Drawing for the job (mm, zero at the part's lowest x, y, z). A direction names the side the tool comes from. Coordinates: 2 decimals unless noted, no trailing zeros. Order: outer loops, then holes, each group sorted by start corner. A loop starts at its lowest first (then second) coordinate and runs counter-clockwise, first axis right, second up. Notation, with made-up numbers: (71, 72) - (114, 72) arc R19 cw to (114, 101) - close; hole circle Ø1 at (23, 44.25). An arc over 180 degrees is marked (long way). Put each result on its own line as item: value. Start each with the question number.
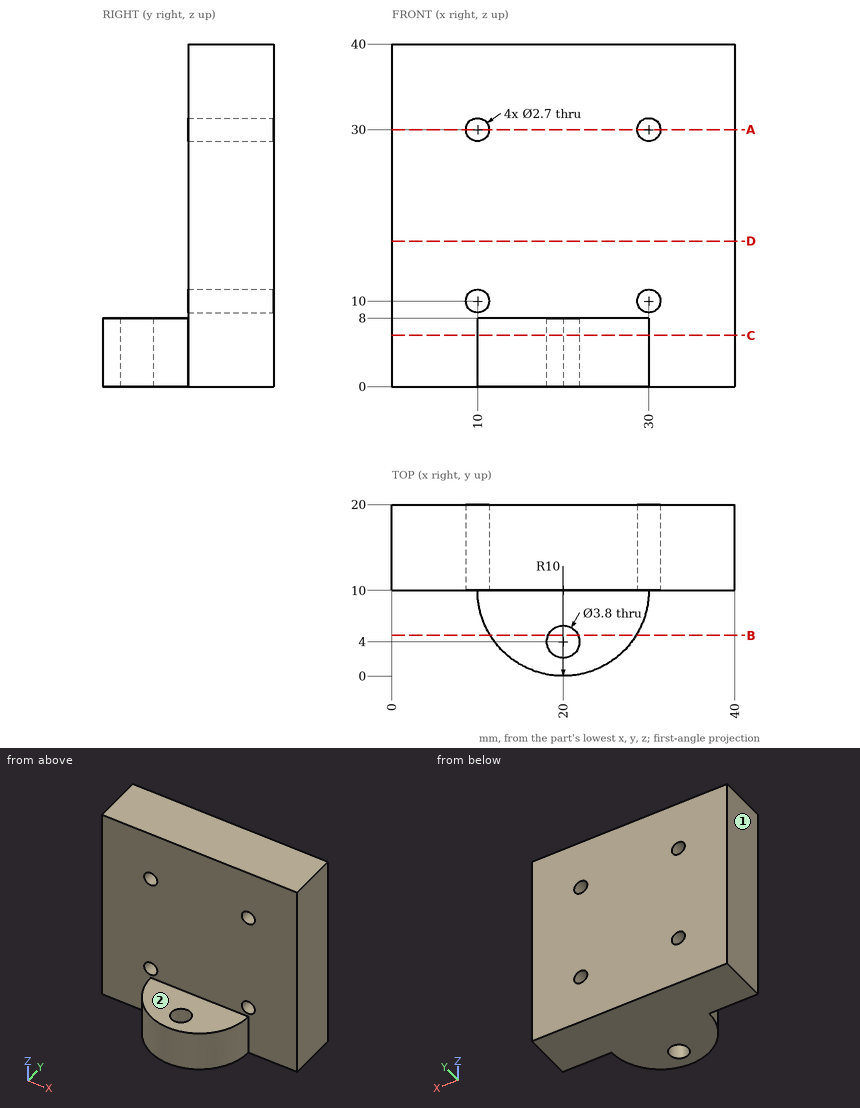
Item 1: Wall check: line 1 along X through (y, z) = (16.25, 30); line 2 along Y through (x, z) = (9, 3); line 3 along Z through (x, y) = (25, 9). Give the ranges that are in metal, low to high.
Item 2: Flat gauge pins, fed straight in: pin 1 Ø3 at (x, z) = (13, 34.5) entering from -Y; pin 2 Ø1.5 at (x, y) = (27, 3.5) entering from +Z. Where does each tip first touch, or does it go through?
Item 3: 3-axis set-ups, long thin cutter, end or side, ignore diameter. For the marked faces 1 and 2: which of +Z, -Z, +X, -X, +Y, -Y reach the whole face in a straight line?
Item 4: Slice it at D-D, the plane z = 17. Give the cut face in (x, y), plus the area to 3 significant figures.
Item 5: Slice it at B-B, the plane y = 4.75. Give the cut face in (x, z).
Item 6: Slice it at C-C, the plane z = 6. Give the cut face in (x, y), plus the area to 3 significant figures.
Item 7: Slice it at A-A, the plane z = 30. Give the cut face in (x, y), plus the area to 3 significant figures.
Here are the results:
1. line 1: x = 0 to 8.65, 11.35 to 28.65, 31.35 to 40
1. line 2: y = 10 to 20
1. line 3: z = 0 to 8
2. pin 1: stops at y = 10
2. pin 2: stops at z = 8
3. face 1: +Z, -Z, -X, +Y, -Y
3. face 2: +Z, +X, -X, -Y
4. outline: (0, 10) - (40, 10) - (40, 20) - (0, 20) - close
4. area: 400 mm^2
5. outline: (11.49, 0) - (18.25, 0) - (18.25, 8) - (11.49, 8) - close; (21.75, 0) - (28.51, 0) - (28.51, 8) - (21.75, 8) - close
6. outline: (0, 10) - (10, 10) arc R10 ccw to (30, 10) - (40, 10) - (40, 20) - (0, 20) - close; hole circle Ø3.8 at (20, 4)
6. area: 546 mm^2
7. outline: (0, 10) - (8.65, 10) - (8.65, 20) - (0, 20) - close; (11.35, 10) - (28.65, 10) - (28.65, 20) - (11.35, 20) - close; (31.35, 10) - (40, 10) - (40, 20) - (31.35, 20) - close
7. area: 346 mm^2
